Here's the drawing with two shaded views (mm, measured from the low corner). I have some questions. Give positions to 0.01 mm unless a question says otherwise; leave off trailing zeros. Write each loop counter-clockwise with the first axis right and the second up, starting at its lowest first coordinate (ties: lowest second). Pieces come first, ordered by that corner, then holes. Notation, with made-up numbers: (41.25, 11.25) - (80.25, 11.25) arc R30 ccw to (80.25, 47.25) - close; hole circle Ø6 at (35.25, 63.25). An arc over 180 degrees is marked (long way). Use one line per item in the form item = value.
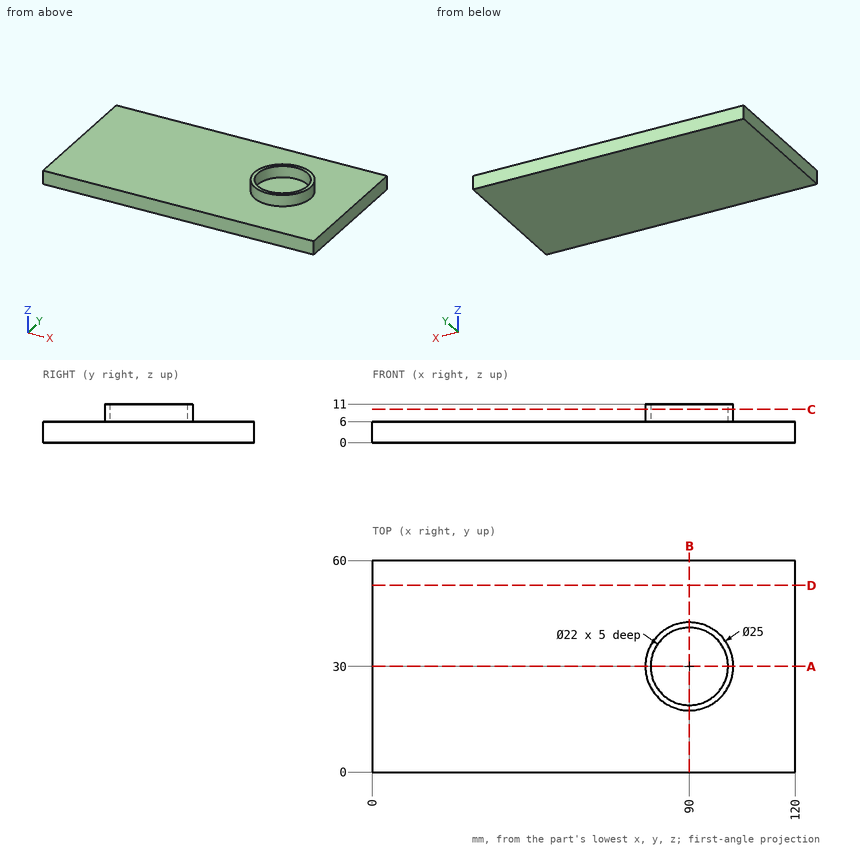
1. Imagine slicing it at A-A, the plane y = 30. List the corners of the cut face in (x, z) for me, and give its area (3 significant figures).
Response values:
outline = (0, 0) - (120, 0) - (120, 6) - (102.5, 6) - (102.5, 11) - (101, 11) - (101, 6) - (79, 6) - (79, 11) - (77.5, 11) - (77.5, 6) - (0, 6) - close
area = 735 mm²
2. Imagine slicing it at D-D, the plane y = 53. List the corners of the cut face in (x, z) for me, and give its area (3 significant figures).
Response values:
outline = (0, 0) - (120, 0) - (120, 6) - (0, 6) - close
area = 720 mm²
3. Imagine slicing it at B-B, the plane x = 90. List the corners of the cut face in (y, z) for me, and give its area (3 significant figures).
Response values:
outline = (0, 0) - (60, 0) - (60, 6) - (42.5, 6) - (42.5, 11) - (41, 11) - (41, 6) - (19, 6) - (19, 11) - (17.5, 11) - (17.5, 6) - (0, 6) - close
area = 375 mm²
4. If I drill on line 1 (Y direction, x = 90, z = 9.7); line 2 (Z direction, x = 26, y = 43); line 3 (X direction, y = 28, z = 6.75), over which ranges is the centre line in solid material (lowest first)? Write a range as from..to.
Response values:
line_1 = 17.5..19, 41..42.5
line_2 = 0..6
line_3 = 77.66..79.18, 100.82..102.34
5. Imagine slicing it at C-C, the plane z = 9.5. List the corners of the cut face in (x, y) for me, and give its area (3 significant figures).
Response values:
outline = circle Ø25 at (90, 30); hole circle Ø22 at (90, 30)
area = 111 mm²
